Here's the drawing with two shaded views (mm, measured from the low corner). I have some questions. Round coordinates to 2 decimals unless told otherwise and drop trailing zeros. Order: outer loops, then holes, each group sorted by start corner. A loop starts at its lowest first (then second) coordinate and runs counter-clockwise, first axis right, second up. Notation, with made-up numbers: (27.5, -5.75) - (32.5, -5.75) arc R17 ccw to (32.5, 24.25) - close; hole circle Ø10 at (40, -38). An arc over 180 degrees is marked (long way). One line per item, written item: value.
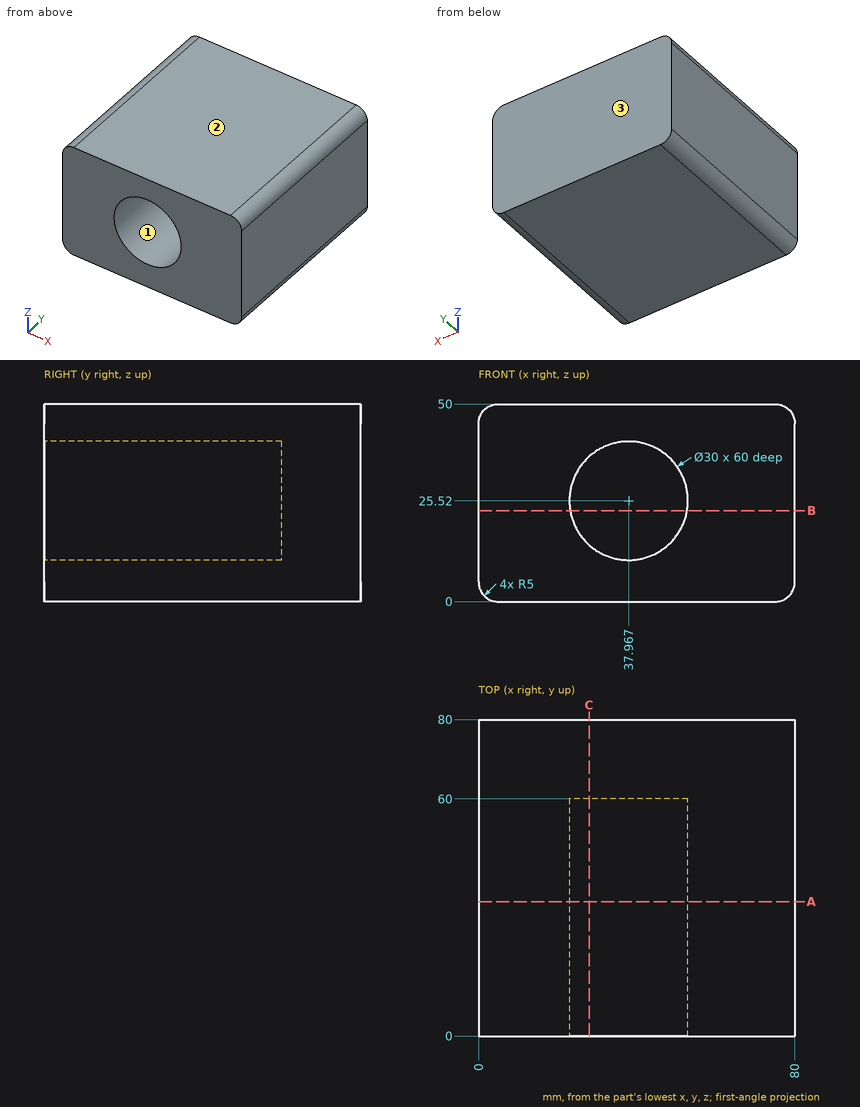
Q1. If we section it at A-A, the plane y = 34: Please give me the cut outline in (x, z), then the cut area to 3 significant figures.
Results list:
outline: (0, 5) arc R5 ccw to (5, 0) - (75, 0) arc R5 ccw to (80, 5) - (80, 45) arc R5 ccw to (75, 50) - (5, 50) arc R5 ccw to (0, 45) - close; hole circle Ø30 at (37.97, 25.52)
area: 3,270 mm²
Q2. If we section it at C-C, the plane x = 28: Please give me the cut outline in (y, z), then the cut area to 4 significant figures.
Results list:
outline: (0, 0) - (80, 0) - (80, 50) - (0, 50) - (0, 36.73) - (60, 36.73) - (60, 14.31) - (0, 14.31) - close
area: 2,655 mm²
Q3. If I drill on line 1 along X through (y, z) = (12.5, 28); line 2 along Y through (x, z) = (44, 23.5); line 3 along X through (y, z) = (13.5, 19.5) (1 decimal), over which ranges is the centre line in solid material (lowest first)?
Results list:
line 1: 0 to 23.17, 52.76 to 80
line 2: 60 to 80
line 3: 0 to 24.2, 51.7 to 80
Q4. We'd pull the mould along Z, two halves only. Please class the marked faces 1, 2 and 3: released by +Z, released by -Z, zero draft, split by the parting line, or undercut.
Results list:
face 1: undercut
face 2: released by +Z
face 3: zero draft
Q5. If we section it at B-B, the plane z = 23: Please give me the cut outline in (x, y) (1 decimal).
Results list:
outline: (0, 0) - (23.2, 0) - (23.2, 60) - (52.8, 60) - (52.8, 0) - (80, 0) - (80, 80) - (0, 80) - close
Q6. Will this pin go through, and if not, where does the flat tip stop? pin 1 (3 mm diameter, centred on x = 39, z = 35, fed in from -Y).
Results list:
pin 1: y = 60
